```python
from build123d import *

# Parameters (mm, degrees)
F0_W     = 65.1499927044
F0_H     = 41.9776812196
F1_DEPTH = 25.4
F2_R     = 2.95
F3_DEPTH = 22.86
F4_DEPTH = 71.30122


with BuildPart() as f1:
    # F0 (on Front) → F1 (new body)
    with BuildSketch(Plane.XZ):
        with Locations((32.5749963522, 20.9888406098)):
            Rectangle(F0_W, F0_H)
    extrude(amount=F1_DEPTH)

    # F2 (on face) → F3, piece 2 (join)
    with BuildSketch(Plane.XZ.offset(25.4)):
        with Locations((38.1691530347, 19.1963799298)):
            Circle(F2_R)
    extrude(amount=F3_DEPTH)

    # F4 (add): a face of the model
    f4_faces = [f1.faces().sort_by_distance(p)[0] for p in [
        (0, -12.7, 20.9888406098),
    ]]


with BuildPart() as f3:
    # F2 (on face) → F3 (new body)
    with BuildSketch(Plane.XZ.offset(25.4)):
        with Locations((-14.9930469653, 17.4420047551)):
            Circle(F2_R)
    extrude(amount=F3_DEPTH)


with BuildPart() as f1_1:
    add(f1.part)

    add(f3.part)  # F4 merges F3
    extrude(f4_faces, amount=F4_DEPTH)


solid = f1_1.part
```
Can you work these out from the model? Positions are in its coordinate system, mm. Coordinates: 2 decimals unless noted, no trailing zeros. Loops run counter-clockwise (first coordinate to the right, second up) from the corner with the lowest first, then second, coordinate; pieces in that order, holes last.
1) Imagine slicing it at A-A on x = 18. List the corners of the cut face in (y, z) for me, plus the area to 3 significant figures.
2) Thinking about a two-plate mould opening in X: for faces 1 (the cylindrical face through (-17.2, -36.7, 19.4)), 2 (the flat face through (-2, -13, 0)), 3 (the flat face through (-71.301, -13, 21)), 4 (the cylindrical face through (39.76, -36.67, 21.68)), which applies, pulls with the +X half, pulls with the -X half, needs draft (parallel to the pull), parting line crosses it, or undercut?
3) I need wall thicknesses on probe 1 along Y at (x, z) = (-59, 14); probe 2 along Z at (x, y) = (-16.5, -29). Which ranges of each line are inside material? Lowest first, please.
4) Imagine slicing it at B-B on z = 27. List the corners of the cut face in (x, y) for me.
5) Imagine slicing it at C-C on y = -31.5. List the corners of the cut face in (x, z) for me, plus the area to 3 significant figures.
6) For pin 1 (12.5 mm diameter, centred on x = 11, z = 26, fed in from -Y), with a flat end and sliding along its axis, tell me the tip position at first contact or that it passes through.
Completed:
1. outline: (-25.4, 0) - (0, 0) - (0, 41.98) - (-25.4, 41.98) - close
1. area: 1,070 mm2
2. face 1: undercut
2. face 2: needs draft
2. face 3: pulls with the -X half
2. face 4: undercut
3. probe 1: y = -25.4 to 0
3. probe 2: z = 14.91 to 19.98
4. outline: (-71.3, -25.4) - (65.15, -25.4) - (65.15, 0) - (-71.3, 0) - close
5. outline: circle Ø5.9 at (-14.99, 17.44); circle Ø5.9 at (38.17, 19.2)
5. area: 54.7 mm2
6. pin 1: stops at y = -25.4
